The listing builds one solid part. Answer for the finished solid, in the listing's coordinates (mm). A direction names the side the tool comes from. Coordinates: 2 decimals unless noted, no trailing zeros. Loops run counter-clockwise (first coordinate to the right, second up) from the corner with the lowest first, then second, coordinate; pieces in that order, holes last. Notation, with made-up numbers: M 12,-29 L 48,-29 A24 ccw 48,0 Z; hole C -28.5,73 d2. An arc over 180 degrees is marked long. Answer as a JSON object with one key per item and string values. Group by question number.
1. Straight lines are drawn through the part: L1, parallel to X at y = -78, z = -29; L2, parallel to Z at x = -67.5, y = -40; L3, parallel to X at y = -146, z = 13. For each, find the intervals that lie inside material, in ascending order.
2. A cutting plane is placed at A-A on x = 57.5. Give the vertices of the cut face in (y, z).
3. For faces 1 (the face through (-40, -14, -14)), 2 (the face through (-32.64, -111.96, -119.6)), 3 (the face through (79.5, -114.81, -122.65)), 4 (the face through (85, -124, -51)), determine the directions among +Z, -Z, +X, -X, +Y, -Y from which every point of the face is accessible in a straight line to the end or side of a thin tool.
4. Given pin 1 (1.5 mm diameter, centred on x = 6, z = -6.5, fed in from +Y); pin 2 (6 mm diameter, centred on x = -50, y = -22.5, fed in from +Z); pin 3 (1 mm diameter, centred on x = -30.5, z = -77.5, fed in from +Y), each flat-ended and moving along its own axis, determine where each tip first touches the part or whether it passes through.
5. Determine the mould class of faces 5 (the face through (57.05, -123.01, -131.41)), 6 (the face through (-85, -100, -88)), 7 (the face through (-57.229, -126.429, -135.058)) for opening direction X: released by +X, released by -X, zero draft, split by the parting line, or undercut.
6. A cutting plane is placed at B-B on x = -57. Give the vertices of the cut face in (y, z).
from build123d import *

# Parameters (mm, degrees)
REVOLVE_THIN1_ANGLE = 270


with BuildPart() as part:
    # Sketch2 → Revolve-Thin1 (revolve)
    with BuildSketch(Plane.XY):
        Polygon((-40, 15), (40, 15), (40, 59), (31.5, 59), (31.5, 104.867188985), (85, 129.814648696), (85, 168), (74.160544448, 168), (65.12148411, 185), (49.11287792, 185), (40.073817581, 168), (36.082423772, 168), (27.043363433, 185), (11.034757243, 185), (1.995696905, 168), (-1.995696905, 168), (-11.034757243, 185), (-27.043363433, 185), (-36.082423772, 168), (-40.073817581, 168), (-49.11287792, 185), (-65.12148411, 185), (-74.160544448, 168), (-85, 168), (-85, 129.814648696), (-31.5, 104.867188985), (-31.5, 59), (-40, 59), align=None)
        Polygon((-35, 20), (35, 20), (35, 54), (26.5, 54), (26.5, 108.052540289), (80, 133), (80, 163), (71.156241353, 163), (62.117181015, 180), (52.117181015, 180), (43.078120676, 163), (33.078120676, 163), (24.039060338, 180), (14.039060338, 180), (5, 163), (-5, 163), (-14.039060338, 180), (-24.039060338, 180), (-33.078120676, 163), (-43.078120676, 163), (-52.117181015, 180), (-62.117181015, 180), (-71.156241353, 163), (-80, 163), (-80, 133), (-26.5, 108.052540289), (-26.5, 54), (-35, 54), align=None, mode=Mode.SUBTRACT)
    revolve(axis=Axis((-156.924897256, 0, 0), (-1, 0, 0)), revolution_arc=REVOLVE_THIN1_ANGLE)


solid = part.part
From the geometry:
{
 "1": {"L1": "x = -31.5 to -26.5, 26.5 to 31.5", "L2": "z = -176.04 to -165.1, -120.72 to -114.89, 114.89 to 120.72, 165.1 to 176.04", "L3": "x = -85 to -80, 80 to 85"},
 "2": {"outline": "M 0,116.99 L 0,122.51 A122.51 ccw long 122.51,0 L 116.99,0 A116.99 cw long Z; M 0,180 L 0,185 A185 ccw long 185,0 L 180,0 A180 cw long Z"},
 "3": {"face 1": "-X", "face 2": "none", "face 3": "+X", "face 4": "+Z, -Z, +X, +Y, -Y"},
 "4": {"pin 1": "stops at y = 176.82", "pin 2": "stops at z = 183.97", "pin 3": "stops at y = 161.87"},
 "5": {"face 5": "undercut", "face 6": "released by -X", "face 7": "zero draft"},
 "6": {"outline": "M 0,116.76 L 0,122.27 A122.27 ccw long 122.27,0 L 116.76,0 A116.76 cw long Z; M 0,180 L 0,185 A185 ccw long 185,0 L 180,0 A180 cw long Z"}
}
